Can you work these out from the model? Positions are in its coordinate system, mm. A direction names the side the tool comes from. Give positions to 0.01 mm unless a question says otherwise; leave off trailing zeros. Loops run counter-clockwise (first coordinate to the right, second up) from the corner with the lowest first, then second, coordinate; pieces in that order, holes last. Notation, with made-up numbers: (-6, 6.5) - (49, 6.5) arc R12 cw to (49, 15.5) - close; hole circle Ø11 at (39.25, 76). An arc over 180 degrees is marked (long way). Write item = value, one per line.
from build123d import *

# Parameters (mm, degrees)
F0_R     = 50
F1_DEPTH = 4
F2_R     = 25
F3_DEPTH = 25
F4_W     = 14
F4_H     = 30
F5_DEPTH = 5


with BuildPart() as f1:
    # F0 (on Top) → F1 (new body)
    with BuildSketch(Plane.XY):
        Circle(F0_R)
    extrude(amount=F1_DEPTH)

    # F2 (on face) → F3 (join)
    with BuildSketch(Plane.XY.offset(4)):
        Circle(F2_R)
    extrude(amount=F3_DEPTH)

    # F4 (on face) → F5 (cut)
    with BuildSketch(Plane(origin=(0, 0, 0), x_dir=(1, 0, 0), z_dir=(0, 0, -1))):
        with Locations((35, 0)):
            Rectangle(F4_W, F4_H)
    extrude(amount=-F5_DEPTH, mode=Mode.SUBTRACT)


solid = f1.part
Q1. Imagine slicing it at B-B, the plane x = 0. Write out the boundary of the cut face in (y, z).
Output:
outline = (-50, 0) - (50, 0) - (50, 4) - (25, 4) - (25, 29) - (-25, 29) - (-25, 4) - (-50, 4) - close
Q2. Which directions (+Z, -Z, +X, -X, +Y, -Y) give clear straight access to the entire face, cutting with the end or side of a thin tool? Please do faces 5 (the flat face through (-22.9, -10.4, 4)), 6 (the flat face through (0, 0, 29)), 7 (the flat face through (35, -15, 2)).
Output:
face_5 = +Z
face_6 = +Z, +X, -X, +Y, -Y
face_7 = +Z, -Z
Q3. We'd pull the mould along X, two halves only. Please class faces 1 (the flat face through (28, 0, 2)), 2 (the cylindrical face through (47.69, 15.02, 1.97)), 3 (the flat face through (-1, 1, 0)), 4 (the flat face through (35, 15, 2)): released by +X, released by -X, zero draft, split by the parting line, or undercut.
Output:
face_1 = undercut
face_2 = split by the parting line
face_3 = zero draft
face_4 = undercut
Q4. Imagine slicing it at D-D, the plane z = 15.75. Write out the boundary of the cut face in (x, y).
Output:
outline = circle Ø50 at (0, 0)
Q5. For pin 1 (10 mm diameter, centred on x = -16.5, z = 12, fed in from -Y); pin 2 (4 mm diameter, centred on x = -0.5, z = 5, fed in from -Y); pin 3 (4 mm diameter, centred on x = 13, z = 5.5, fed in from -Y), each with a flat end and sliding along its axis, tell me the tip position at first contact or that it passes through.
Output:
pin_1 = -22.2
pin_2 = -50
pin_3 = -48.62
Q6. I need wall thicknesses on L1, parallel to Z at x = 26.5, y = -19; L2, parallel to Y at x = 28.5, z = 3.5; L3, parallel to Y at x = -3, z = 24.5. Which ranges of each line are inside material? Lowest first, please.
Output:
L1 = 0 to 4
L2 = -41.08 to -15, 15 to 41.08
L3 = -24.82 to 24.82
Q7. Imagine slicing it at A-A, the plane y = 0. Write out the boundary of the cut face in (x, z), then the cut area to 3 significant figures.
Output:
outline = (-50, 0) - (28, 0) - (28, 4) - (25, 4) - (25, 29) - (-25, 29) - (-25, 4) - (-50, 4) - close; (42, 0) - (50, 0) - (50, 4) - (42, 4) - close
area = 1,590 mm2
Q8. Imagine slicing it at C-C, the plane y = 21. Write out the boundary of the cut face in (x, z).
Output:
outline = (-45.38, 0) - (45.38, 0) - (45.38, 4) - (13.56, 4) - (13.56, 29) - (-13.56, 29) - (-13.56, 4) - (-45.38, 4) - close
